from build123d import *

# Parameters (mm, degrees)
SKETCH_3_OUTSIDE_W       = 271.478
SKETCH_3_OUTSIDE_H       = 131.478
SKETCH_3_OUTSIDE_W_2     = 220
SKETCH_3_OUTSIDE_H_2     = 40
CUT_EXTRUDE_1_DEPTH      = 41
CUT_EXTRUDE_1_DEPTH_BACK = 41
SKETCH_4_R               = 14
SKETCH_4_W               = 25
SKETCH_4_H               = 9
CUT_EXTRUDE_2_DEPTH      = 41
SKETCH_5_R               = 6.5
CUT_EXTRUDE_3_DEPTH      = 48


with BuildPart() as part:
    # 草圖1 → 旋轉1 (revolve)
    with BuildSketch(Plane.XY):
        with BuildLine():
            Line((29.047375097, 27.5), (90, 27.5))
            Line((90, 27.5), (130, 16))
            Line((130, 16), (180, 16))
            Line((180, 16), (180, 0))
            Line((180, 0), (-40, 0))
            ThreePointArc((-40, 0), (-14.800422226, 37.161102001), (29.047375097, 27.5))
        make_face()
    revolve(axis=Axis((-119.807750387, 0, 0), (1, 0, 0)))

    # 草圖3 outside → 除料-伸長1 (cut, two sides)
    with BuildSketch(Plane(origin=(0, 0, 0), x_dir=(1, 0, 0), z_dir=(0, 1, 0))) as cut_extrude_1_sk:
        with Locations((70, 0)):
            Rectangle(SKETCH_3_OUTSIDE_W, SKETCH_3_OUTSIDE_H)
        with Locations((70, 0)):
            Rectangle(SKETCH_3_OUTSIDE_W_2, SKETCH_3_OUTSIDE_H_2, mode=Mode.SUBTRACT)
    extrude(amount=CUT_EXTRUDE_1_DEPTH, mode=Mode.SUBTRACT)
    extrude(cut_extrude_1_sk.sketch, amount=-CUT_EXTRUDE_1_DEPTH_BACK, mode=Mode.SUBTRACT)

    # 草圖4 → 除料-伸長2 (cut, through all)
    with BuildSketch(Plane.XY.offset(20)):
        Circle(SKETCH_4_R)
        with Locations((167.5, 11.5)):
            Rectangle(SKETCH_4_W, SKETCH_4_H)
        with Locations((167.5, -11.5)):
            Rectangle(SKETCH_4_W, SKETCH_4_H)
    extrude(amount=-CUT_EXTRUDE_2_DEPTH, mode=Mode.SUBTRACT)

    # 草圖5 → 除料-伸長3 (cut, through all)
    with BuildSketch(Plane(origin=(0, 7, 0), x_dir=(1, 0, 0), z_dir=(0, 1, 0))):
        with Locations((168, 0)):
            Circle(SKETCH_5_R)
    extrude(amount=-CUT_EXTRUDE_3_DEPTH, mode=Mode.SUBTRACT)


solid = part.part
Geometry check sheet. Reference: the model listing, model coordinates, mm. A direction names the side the tool comes from. Round coordinates to 2 decimals unless told otherwise and drop trailing zeros. Write each loop counter-clockwise with the first axis right and the second up, starting at its lowest first coordinate (ties: lowest second). Pieces come first, ordered by that corner, then holes. Notation, with made-up numbers: (-7.5, 79.5) - (48.5, 79.5) arc R15 ccw to (48.5, 107.5) - close; hole circle Ø9 at (-34, 25.5). An arc over 180 degrees is marked (long way). One line per item, written item: value.
1. Cross-section at A-A on y = 0. Record the boundary of the cut face in (x, z), and give its area (3 significant figures).
The answers:
outline: (-34.64, -20) - (-14, -20) - (-14, 20) - (-34.64, 20) arc R40 ccw to start; (14, -20) - (116.09, -20) - (130, -16) - (180, -16) - (180, 16) - (130, 16) - (116.09, 20) - (14, 20) - close; hole circle Ø13 at (168, 0)
area: 7,020 mm^2
2. Mould release check, pull along X, two halves, no side actions. Record for faces 1 (the face through (161.506, 0.098, -0.286)), 2 (the face through (144.239, -15.985, 0.703)), 3 (the face through (119.169, -19.095, 0.84)): released by +X, released by -X, zero draft, split by the parting line, or undercut.
The answers:
face 1: undercut
face 2: zero draft
face 3: released by +X
3. Cross-section at B-B on z = 0. Record the boundary of the cut face in (x, y), and give its area (3 significant figures).
The answers:
outline: (29.05, -27.5) - (90, -27.5) - (130, -16) - (155, -16) - (155, -7) - (161.5, -7) - (161.5, 7) - (155, 7) - (155, 16) - (130, 16) - (90, 27.5) - (29.05, 27.5) arc R40 ccw (long way) to start; (174.5, -7) - (180, -7) - (180, 7) - (174.5, 7) - close; hole circle Ø28 at (0, 0)
area: 10,100 mm^2
4. Scan lines: L1, parallel to X at y = 0.5, z = 0; L2, parallel to X at y = -3.5, z = 3; L3, parallel to Z at x = 168, y = 0. Record each from-to range of solid material in increasing order.
The answers:
L1: x = -40 to -13.99, 13.99 to 161.5, 174.5 to 180
L2: x = -39.73 to -13.56, 13.56 to 162.23, 173.77 to 180
L3: z = -16 to -6.5, 6.5 to 16
5. Set-up check for faces 4 (the face through (60, 27.5, -0.3)), 5 (the face through (162, 7, 3)), 6 (the face through (155, -11, 0)): record each of +Z, -Z, +X, -X, +Y, -Y from which the full face is reachable in a straight line by a thin tool's end or side.
The answers:
face 4: +X, +Y
face 5: +Z, -Z, +X, +Y
face 6: +Z, -Z, +X, -Y
6. Depth check by flat-ended pin: pin 1 Ø6 at (x, z) = (130.5, -3) entering from -Y; pin 2 Ø6 at (y, z) = (8.5, 10.5) entering from +X; pin 3 Ø17 at (x, z) = (168, 0) entering from -Y; pin 4 Ø20 at (x, z) = (173.5, -7) entering from +Y. Enter the tip coordinate at first touch or a pass-through.
The answers:
pin 1: stops at y = -16.55
pin 2: stops at x = 180
pin 3: stops at y = -7
pin 4: stops at y = 7
7. Cross-section at C-C on x = 168. Record the boundary of the cut face in (y, z), and give its area (3 significant figures).
The answers:
outline: (-7, -14.39) arc R16 ccw to (7, -14.39) - (7, -6.5) - (-7, -6.5) - close; (-7, 6.5) - (7, 6.5) - (7, 14.39) arc R16 ccw to (-7, 14.39) - close
area: 251 mm^2
8. Cross-section at D-D on x = 0. Record the boundary of the cut face in (y, z), and give its area (3 significant figures).
The answers:
outline: (-34.64, -20) - (-14, -20) - (-14, 20) - (-34.64, 20) arc R40 ccw to start; (14, -20) - (34.64, -20) arc R40 ccw to (34.64, 20) - (14, 20) - close
area: 1,940 mm^2
